Read the model definition and answer for the solid it produces. Units are mm, in the model's axes. Face numbers are marked on the shaded views. A direction names the side the tool comes from. Give positions to 0.01 mm unless a question says otherwise; leave off trailing zeros. Write each loop counter-clockwise with the first axis right and the second up, starting at its lowest first coordinate (ties: lowest second). Pieces come first, ordered by that corner, then holes. Notation, with made-up numbers: (5.25, -33) -> (24.25, -33) arc R10 ccw to (24.25, -17) -> close; hole circle Ø3 at (83.25, 83.25). An arc over 180 degrees is marked (long way). Write item = value, one per line.
from build123d import *

# Parameters (mm, degrees)
SKETCH_1_W                   = 20
SKETCH_1_H                   = 75
EXTRUDE_1_DEPTH              = 6
SKETCH_2_W                   = 6
SKETCH_2_H                   = 75
EXTRUDE_2_DEPTH              = 20
SKETCH_3_W                   = 20
SKETCH_3_H                   = 75
EXTRUDE_3_DEPTH              = 8.1
SKETCH_4_W                   = 14.1
SKETCH_4_H                   = 75
EXTRUDE_4_DEPTH              = 35
HOLE_WIZARD_M6_1_D           = 6.6
HOLE_WIZARD_M6_1_CBORE_D     = 11
HOLE_WIZARD_M6_1_CBORE_DEPTH = 6.4
SKETCH_9_R                   = 6
CUT_EXTRUDE_1_DEPTH          = 2
HOLE_WIZARD_M3_1_D           = 2.5
HOLE_WIZARD_M3_1_DEPTH       = 10.1
HOLE_WIZARD_M3_1_TIP         = 0.751075774
SKETCH_15_W                  = 8
SKETCH_15_H                  = 75
CUT_EXTRUDE_3_DEPTH          = 1
HOLE_WIZARD_M5_1_D           = 5.5
HOLE_WIZARD_M5_1_CBORE_D     = 10
HOLE_WIZARD_M5_1_CBORE_DEPTH = 5.4
HOLE_WIZARD_M6_1_2_D         = 5
HOLE_WIZARD_M6_1_2_DEPTH     = 15
HOLE_WIZARD_M6_1_2_TIP       = 1.502151548
HOLE_WIZARD_M5_2_D           = 5.5
HOLE_WIZARD_M5_2_CBORE_D     = 10
HOLE_WIZARD_M5_2_CBORE_DEPTH = 5.4
SKETCH_24_W                  = 10
SKETCH_24_H                  = 75
CUT_EXTRUDE_4_DEPTH          = 1
SKETCH_25_W                  = 13
SKETCH_25_H                  = 12.5
CUT_EXTRUDE_5_DEPTH          = 15.1


with BuildPart() as part:
    # 草图1 → 凸台-拉伸1 (new body)
    with BuildSketch(Plane.XY):
        with Locations((10, 37.5)):
            Rectangle(SKETCH_1_W, SKETCH_1_H)
    extrude(amount=EXTRUDE_1_DEPTH)

    # 草图2 → 凸台-拉伸2 (add)
    with BuildSketch(Plane.ZY):
        with Locations((3, 37.5)):
            Rectangle(SKETCH_2_W, SKETCH_2_H)
    extrude(amount=EXTRUDE_2_DEPTH)

    # 草图3 → 凸台-拉伸3 (add)
    with BuildSketch(Plane.XY.offset(6)):
        with Locations((-10, 37.5)):
            Rectangle(SKETCH_3_W, SKETCH_3_H)
    extrude(amount=EXTRUDE_3_DEPTH)

    # 草图4 → 凸台-拉伸4 (add)
    with BuildSketch(Plane.ZY.offset(20)):
        with Locations((7.05, 37.5)):
            Rectangle(SKETCH_4_W, SKETCH_4_H)
    extrude(amount=EXTRUDE_4_DEPTH)

    # Hole Wizard M6 _1 (through all)
    with Locations(Plane(origin=(0, 0, 0), x_dir=(-1, 0, 0), z_dir=(0, 0, -1))):
        with Locations((18, 37.5)):
            CounterBoreHole(HOLE_WIZARD_M6_1_D / 2, HOLE_WIZARD_M6_1_CBORE_D / 2, HOLE_WIZARD_M6_1_CBORE_DEPTH)

    # 草图9 → 切除-拉伸1 (cut)
    with BuildSketch(Plane.XY.offset(14.1)):
        with Locations((-18, 37.5)):
            Circle(SKETCH_9_R)
    extrude(amount=-CUT_EXTRUDE_1_DEPTH, mode=Mode.SUBTRACT)

    # M3 螺纹孔1
    with Locations(Plane.XY.offset(14.1)):
        with Locations((-4, 7.5), (-4, 67.5)):
            Hole(HOLE_WIZARD_M3_1_D / 2, depth=HOLE_WIZARD_M3_1_DEPTH)
            with Locations((0, 0, -(HOLE_WIZARD_M3_1_DEPTH + HOLE_WIZARD_M3_1_TIP / 2))):  # 118° drill point
                Cone(0, HOLE_WIZARD_M3_1_D / 2, HOLE_WIZARD_M3_1_TIP, mode=Mode.SUBTRACT)

    # 草图15 → 切除-拉伸3 (cut)
    with BuildSketch(Plane.XY.offset(14.1)):
        with Locations((-46, 37.5)):
            Rectangle(SKETCH_15_W, SKETCH_15_H)
    extrude(amount=-CUT_EXTRUDE_3_DEPTH, mode=Mode.SUBTRACT)

    # M5 六角凹头螺钉的柱形沉头孔1 (through all)
    with Locations(Plane(origin=(0, 0, 0), x_dir=(-1, 0, 0), z_dir=(0, 0, -1))):
        with Locations((46, 52.5), (46, 22.5)):
            CounterBoreHole(HOLE_WIZARD_M5_1_D / 2, HOLE_WIZARD_M5_1_CBORE_D / 2, HOLE_WIZARD_M5_1_CBORE_DEPTH)

    # Hole Wizard M6 _1 2
    with Locations(Plane.XY.offset(14.1)):
        with Locations((-33, 37.5)):
            Hole(HOLE_WIZARD_M6_1_2_D / 2, depth=HOLE_WIZARD_M6_1_2_DEPTH)
            with Locations((0, 0, -(HOLE_WIZARD_M6_1_2_DEPTH + HOLE_WIZARD_M6_1_2_TIP / 2))):  # 118° drill point
                Cone(0, HOLE_WIZARD_M6_1_2_D / 2, HOLE_WIZARD_M6_1_2_TIP, mode=Mode.SUBTRACT)

    # M5 六角凹头螺钉的柱形沉头孔2 (through all)
    with Locations(Plane.XY.offset(14.1)):
        with Locations((-33, 57.5), (-33, 17.5)):
            CounterBoreHole(HOLE_WIZARD_M5_2_D / 2, HOLE_WIZARD_M5_2_CBORE_D / 2, HOLE_WIZARD_M5_2_CBORE_DEPTH)

    # 草图24 → 切除-拉伸4 (cut)
    with BuildSketch(Plane(origin=(0, 0, 0), x_dir=(-1, 0, 0), z_dir=(0, 0, -1))):
        with Locations((33, 37.5)):
            Rectangle(SKETCH_24_W, SKETCH_24_H)
    extrude(amount=-CUT_EXTRUDE_4_DEPTH, mode=Mode.SUBTRACT)

    # 草图25 → 切除-拉伸5 (cut, through all)
    with BuildSketch(Plane.XY.offset(14.1)):
        with Locations((-48.5, 6.25)):
            Rectangle(SKETCH_25_W, SKETCH_25_H)
        with Locations((-48.5, 68.75)):
            Rectangle(SKETCH_25_W, SKETCH_25_H)
    extrude(amount=-CUT_EXTRUDE_5_DEPTH, mode=Mode.SUBTRACT)


solid = part.part
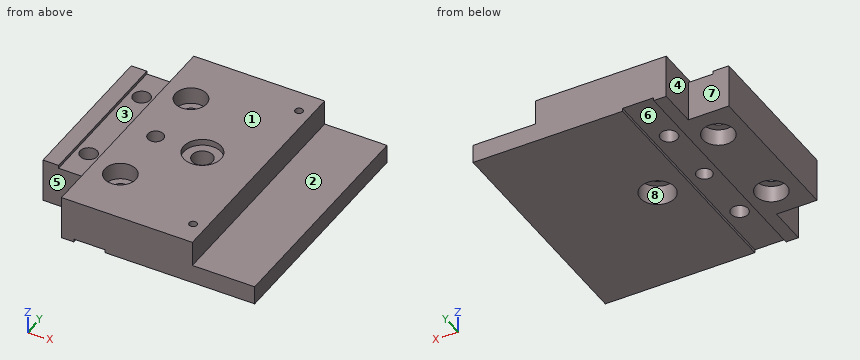
(1) For a pull along Y with two mould halves and no side action, classify the marked faces 5, 6, 7 and 8 as released by +Y, released by -Y, zero draft, split by the parting line, or undercut.
Checks:
face_5 = released by -Y
face_6 = zero draft
face_7 = released by +Y
face_8 = undercut
(2) Consider L1, parallel to Y at x = -46, z = 2.05; L2, parallel to Y at x = -46, z = 8.5; L3, parallel to Y at x = -33, z = 9.8. Determine where each line is inside the solid, lowest interval first.
Checks:
L1 = 12.5 to 17.5, 27.5 to 47.5, 57.5 to 62.5
L2 = 12.5 to 19.75, 25.25 to 49.75, 55.25 to 62.5
L3 = 0 to 12.5, 22.5 to 35, 40 to 52.5, 62.5 to 75
(3) The part is cut by section C-C on y = 58.5. Determine the outline of the cut face in (x, z).
Checks:
outline = (-55, 0) -> (-38, 0) -> (-38, 1) -> (-35.56, 1) -> (-35.56, 8.7) -> (-37.9, 8.7) -> (-37.9, 14.1) -> (-42, 14.1) -> (-42, 13.1) -> (-50, 13.1) -> (-50, 14.1) -> (-55, 14.1) -> close; (-30.44, 1) -> (-28, 1) -> (-28, 0) -> (20, 0) -> (20, 6) -> (0, 6) -> (0, 14.1) -> (-28.1, 14.1) -> (-28.1, 8.7) -> (-30.44, 8.7) -> close
(4) The part is cut by section A-A on x = -33. Determine the outline of the cut face in (y, z).
Checks:
outline = (0, 1) -> (14.75, 1) -> (14.75, 8.7) -> (12.5, 8.7) -> (12.5, 14.1) -> (0, 14.1) -> close; (20.25, 1) -> (35, 1) -> (35, 14.1) -> (22.5, 14.1) -> (22.5, 8.7) -> (20.25, 8.7) -> close; (40, 1) -> (54.75, 1) -> (54.75, 8.7) -> (52.5, 8.7) -> (52.5, 14.1) -> (40, 14.1) -> close; (60.25, 1) -> (75, 1) -> (75, 14.1) -> (62.5, 14.1) -> (62.5, 8.7) -> (60.25, 8.7) -> close
(5) The part is cut by section D-D on x = -17.5. Determine the outline of the cut face in (y, z), plus the area to 3 significant figures.
Checks:
outline = (0, 0) -> (32.02, 0) -> (32.02, 6.4) -> (34.24, 6.4) -> (34.24, 12.1) -> (31.52, 12.1) -> (31.52, 14.1) -> (0, 14.1) -> close; (40.76, 6.4) -> (42.98, 6.4) -> (42.98, 0) -> (75, 0) -> (75, 14.1) -> (43.48, 14.1) -> (43.48, 12.1) -> (40.76, 12.1) -> close
area = 926 mm²
(6) A tool of negligible diameter and unlimited length cuts with its end or side. For the marked faces 1, 2, 3 and 4, from which of +Z, -Z, +X, -X, +Y, -Y can it reach the whole face along a straight path? Write none if from no direction.
Checks:
face_1 = +Z, +X, -X, +Y, -Y
face_2 = +Z, +X, +Y, -Y
face_3 = +Z, +Y, -Y
face_4 = +Z
(7) Given P1, Ø9.5, axis at x = -18, y = 37.5, coming from the +Z side; P2, Ø4, axis at y = 22.5, z = 10, coming from the +X side; P3, Ø8, axis at x = -46, y = 52.5, coming from the -Z side, each flat-ended and moving along its own axis, determine where each tip first touches the part or whether it passes through.
Checks:
P1 = 12.1
P2 = 0
P3 = 5.4
(8) The part is cut by section B-B on x = -46. Determine the outline of the cut face in (y, z), plus the area to 3 significant figures.
Checks:
outline = (12.5, 0) -> (17.5, 0) -> (17.5, 5.4) -> (19.75, 5.4) -> (19.75, 13.1) -> (12.5, 13.1) -> close; (25.25, 5.4) -> (27.5, 5.4) -> (27.5, 0) -> (47.5, 0) -> (47.5, 5.4) -> (49.75, 5.4) -> (49.75, 13.1) -> (25.25, 13.1) -> close; (55.25, 5.4) -> (57.5, 5.4) -> (57.5, 0) -> (62.5, 0) -> (62.5, 13.1) -> (55.25, 13.1) -> close
area = 462 mm²
